The model under review builds one solid part; all positions refer to its coordinate system, in mm. A direction names the side the tool comes from. Coordinates: 2 decimals unless noted, no trailing zeros. Loops run counter-clockwise (first coordinate to the right, second up) from the corner with the lowest first, then second, coordinate; pieces in that order, holes last. Notation, with made-up numbers: M -23,50.5 L -11,50.5 A6 ccw -11,56.5 Z; hole C 0,2.25 d8. An arc over 180 degrees is marked long. Write item = value, one per line. Start each with the question number.
Q1. We need section D-D on y = -15. Give the boundary of the cut face in (x, z), and give its area (3 significant figures).
Q2. Wall thickness on probe 1 along Y at (x, z) = (25.4, 5); probe 2 along X at (y, z) = (-9.25, 5); probe 3 along Y at (x, z) = (44.45, 8): over which ranges is each line inside the solid? List them lowest first.
Q3. We need section C-C on z = 12. Give the boundary of the cut face in (x, y), and give its area (3 significant figures).
Q4. Clearance check with flat-ended pins moving along their axes: pin 1 Ø4 at (y, z) = (-8, 19) entering from +X; pin 2 Ø1.5 at (y, z) = (-19.5, 12) entering from +X. State where each tip first meets the part, or that it passes through.
Q5. We need section B-B on z = 39.5. Give the boundary of the cut face in (x, y), and give its area (3 significant figures).
Q6. We need section A-A on x = 44.45. Give the boundary of the cut face in (y, z), and give its area (3 significant figures).
Q7. For faces 1 (the face through (6, -19.05, 38)), 2 (the face through (35, -13, 12.7)), 3 (the face through (20.36, -16.6, 6.44)), list the 3-axis set-ups (+Z, -Z, +X, -X, +Y, -Y) from which the entire face can be reached by the end or side of a thin tool; tool diameter is ignored.
from build123d import *

# Parameters (mm, degrees)
F1_DEPTH = 25.4
F3_DEPTH = 12.7
F4_R     = 6.35
F5_DEPTH = 25.4


# Not quite as in the source:
# - ends of sketch curves that miss each other by under 0.0002 mm in the source are joined


with BuildPart() as f1:
    # F0 (on Front) → F1 (new body)
    with BuildSketch(Plane.XZ):
        Polygon((0, 44.45), (0, 0), (57.15, 0), (57.15, 12.7), (12.7, 12.7), (12.7, 44.45), align=None)
    extrude(amount=F1_DEPTH)

    # F2 (on face) → F3 (cut)
    with BuildSketch(Plane.YZ.offset(12.7)):
        with BuildLine():
            Line((-12.7, 31.75), (-19.05, 31.75))
            ThreePointArc((-19.05, 31.75), (-12.7, 25.4), (-6.35, 31.75))
            Line((-6.35, 31.75), (-12.7, 31.75))
        make_face()
        with BuildLine():
            Line((-19.05, 44.45), (-19.05, 31.75))
            ThreePointArc((-19.05, 31.75), (-12.732894977, 38.0999147963), (-6.3503408124, 31.8157890712))
            Line((-6.3503408124, 31.8157890712), (-6.4812591328, 44.45))
            Line((-6.4812591328, 44.45), (-19.05, 44.45))
        make_face()
        with BuildLine():
            ThreePointArc((-6.3503408124, 31.8157890712), (-12.732894977, 38.0999147963), (-19.05, 31.75))
            Line((-19.05, 31.75), (-12.7, 31.75))
            Line((-12.7, 31.75), (-6.35, 31.75))
            ThreePointArc((-6.35, 31.75), (-6.3500852037, 31.782894977), (-6.3503408124, 31.8157890712))
        make_face()
        with BuildLine():
            ThreePointArc((-25.4, 38.1), (-23.5401280605, 42.5901280605), (-19.05, 44.45))
            Line((-19.05, 44.45), (-25.4, 44.45))
            Line((-25.4, 44.45), (-25.4, 38.1))
        make_face()
        with BuildLine():
            Line((0, 44.45), (-6.4812591328, 44.45))
            ThreePointArc((-6.4812591328, 44.45), (-1.9444866031, 42.597935184), (0, 38.1))
            Line((0, 38.1), (0, 44.45))
        make_face()
    extrude(amount=-F3_DEPTH, mode=Mode.SUBTRACT)

    # F4 (on face) → F5 (cut)
    with BuildSketch(Plane.XY.offset(12.7)):
        with Locations((25.4, -12.7384394317)):
            Circle(F4_R)
        with Locations((44.45, -12.5940097496)):
            Circle(F4_R)
        with BuildLine():
            ThreePointArc((48.39091748, 0), (54.5541990648, -4.3642287783), (57.15, -11.4560797516))
            Line((57.15, -11.4560797516), (57.15, 0))
            Line((57.15, 0), (48.39091748, 0))
        make_face()
        with BuildLine():
            Line((57.15, -25.4), (57.15, -16.1034604334))
            ThreePointArc((57.15, -16.1034604334), (55.1119721944, -21.4757258052), (50.91496557, -25.4))
            Line((50.91496557, -25.4), (57.15, -25.4))
        make_face()
    extrude(amount=-F5_DEPTH, mode=Mode.SUBTRACT)


solid = f1.part
Returned:
q1.outline = M 0,0 L 19.47,0 L 19.47,12.7 L 12.7,12.7 L 12.7,25.83 L 0,25.83 Z; M 31.33,0 L 38.57,0 L 38.57,12.7 L 31.33,12.7 Z; M 50.33,0 L 57.15,0 L 57.15,12.7 L 50.33,12.7 Z
q1.area = 593 mm^2
q2.probe_1 = -25.4 to -19.09, -6.39 to 0
q2.probe_2 = 0 to 20.09, 30.71 to 39.05, 49.85 to 56.85
q2.probe_3 = -25.4 to -18.94, -6.24 to 0
q3.outline = M 0,-25.4 L 50.91,-25.4 A12.7 ccw 57.15,-16.1 L 57.15,-11.46 A12.7 ccw 48.39,0 L 0,0 Z; hole C 25.4,-12.74 d12.7; hole C 44.45,-12.59 d12.7
q3.area = 1,150 mm^2
q4.pin_1 = 12.7
q4.pin_2 = 56.5
q5.outline = M 0,-25.24 L 12.7,-25.24 L 12.7,-19.05 L 0,-19.05 Z; M 0,-6.43 L 12.7,-6.43 L 12.7,-0.18 L 0,-0.18 Z
q5.area = 158 mm^2
q6.outline = M -25.4,0 L -18.94,0 L -18.94,12.7 L -25.4,12.7 Z; M -6.24,0 L 0,0 L 0,12.7 L -6.24,12.7 Z
q6.area = 161 mm^2
q7.face_1 = +Z, +X, -X
q7.face_2 = +Z, +X, +Y, -Y
q7.face_3 = +Z, -Z
